Could you check a few things on this model? Use its own coordinates, in mm. Face numbers are marked on the shaded views. A direction names the side the tool comes from. Coordinates: 2 decimals unless noted, no trailing zeros. Loops run counter-clockwise (first coordinate to the right, second up) from the corner with the lowest first, then second, coordinate; pieces in that order, holes last.
1) If I drill on line 1 along X through (y, z) = (8, -12); line 2 along X through (y, z) = (5, -10.5); line 3 along Z through (x, y) = (14, 8.25), over which ranges is the centre line in solid material (lowest first)?
2) Imagine slicing it at C-C on x = -5. Please give me the cut outline in (y, z), plus the area to 3 significant figures.
3) For the marked faces 4 and 5, which set-ups out of +Z, -Z, +X, -X, +Y, -Y let a thin tool reach every point of the face, with its end or its side?
4) Imagine slicing it at B-B on x = -29.8. Please give me the cut outline in (y, z), plus the area to 3 significant figures.
5) Will these pins go through, and if not, where does the flat tip stop? P1, Ø1.4, axis at y = 8, z = -17.5, coming from the -X side; P2, Ø0.9, axis at x = -29.5, y = 1.5, coming from the +Z side; P3, Ø1, axis at x = 2, z = -18, coming from the +Y side.
6) Imagine slicing it at A-A on z = -7.6. Please give me the cut outline in (x, y), plus the area to 3 significant figures.
7) Imagine slicing it at D-D on z = 6.5. Please give me the cut outline in (x, y), plus the area to 3 significant figures.
8) Thinking about a two-plate mould opening in Z: for the marked faces 1, 2 and 3, which applies, released by +Z, released by -Z, zero draft, split by the parting line, or undercut?
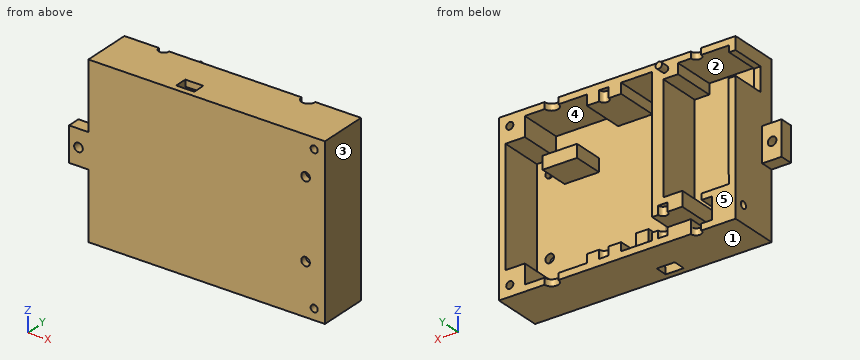
```python
from build123d import *

# Parameters (mm, degrees)
SKETCH_1_W            = 55
SKETCH_1_H            = 39
EXTRUDE_1_DEPTH       = 11.5
SHELL_1_T             = -1.5
SKETCH_2_R            = 1.6
SKETCH_2_R_2          = 1.2
SKETCH_2_W            = 4.2
SKETCH_2_H            = 2.9
CUT_EXTRUDE_1_DEPTH   = 50.086658065
SKETCH_3_W            = 0.1
SKETCH_3_H            = 20.6
SKETCH_3_W_2          = 9
SKETCH_3_H_2          = 1.7
SKETCH_3_W_3          = 8
SKETCH_3_H_3          = 1.95
SKETCH_3_H_4          = 2.4
SKETCH_3_W_4          = 4.5
SKETCH_3_H_5          = 4.5
EXTRUDE_2_DEPTH       = 10
CUT_EXTRUDE_START     = -1.5
SKETCH_4_R            = 1.1
CUT_EXTRUDE_2_DEPTH   = 36
SKETCH_5_R            = 1.1
CUT_EXTRUDE_3_DEPTH   = 7
EXTRUDE_3_DEPTH       = 1.5
EXTRUDE_3_DEPTH_BACK  = 1.5
SKETCH_6_W            = 3
SKETCH_6_H            = 3
SKETCH_6_W_2          = 4.5
SKETCH_6_H_2          = 8
SKETCH_7_R            = 1
SKETCH_7_R_2          = 0.825
CUT_EXTRUDE_4_DEPTH   = 40.198214245
SKETCH_8_R            = 1
CUT_EXTRUDE_5_DEPTH   = 39.784661917
CUT_EXTRUDE_6_REACH   = 61.477
SKETCH_9_R            = 0.825
SKETCH_10_W           = 8
SKETCH_10_H           = 3
F_3MM_4_DEPTH         = 7
CUT_EXTRUDE_4_2_REACH = 61.477
SKETCH_11_W           = 5.5
SKETCH_11_H           = 8
SKETCH_12_R           = 0.75
EXTRUDE_5_DEPTH       = 2


with BuildPart() as part:
    # 草图1 → 凸台-拉伸1 (new body)
    with BuildSketch(Plane(origin=(0, 0, 0), x_dir=(1, 0, 0), z_dir=(0, 1, 0))):
        Rectangle(SKETCH_1_W, SKETCH_1_H)
    extrude(amount=EXTRUDE_1_DEPTH)

    # 抽壳1
    shell_1_openings = [part.faces().sort_by_distance(p)[0] for p in [
        (0, 11.5, 0),
    ]]
    offset(amount=SHELL_1_T, openings=shell_1_openings, kind=Kind.INTERSECTION)

    # 草图2 → 切除-拉伸1 (cut, through all)
    with BuildSketch(Plane(origin=(0, 0, -19.5), x_dir=(-1, 0, 0), z_dir=(0, 0, -1))):
        with Locations((-15.3, 11.5)):
            Circle(SKETCH_2_R)
        with Locations((18.3, 11.5)):
            Circle(SKETCH_2_R_2)
        with Locations((6, 2.85)):
            Rectangle(SKETCH_2_W, SKETCH_2_H)
    extrude(amount=-CUT_EXTRUDE_1_DEPTH, mode=Mode.SUBTRACT)

    # 草图3 → 凸台-拉伸2 (add)
    with BuildSketch(Plane(origin=(0, 1.5, 0), x_dir=(1, 0, 0), z_dir=(0, 1, 0))):
        Polygon((-10.7, 9.6), (-10.7, -15.6), (-14.1, -15.6), (-14.1, -18), (-10.7, -18), (-8.1, -18), (-8.1, 13), (-15.1, 13), (-15.1, 9.6), align=None)
        with Locations((-25.95, -0.7)):
            Rectangle(SKETCH_3_W, SKETCH_3_H)
        with Locations((-12.6, 17.15)):
            Rectangle(SKETCH_3_W_2, SKETCH_3_H_2)
        with Locations((3.1, 17.025)):
            Rectangle(SKETCH_3_W_3, SKETCH_3_H_3)
        with Locations((3.1, -16.8)):
            Rectangle(SKETCH_3_W_3, SKETCH_3_H_4)
        with Locations((23.75, 15.75)):
            Rectangle(SKETCH_3_W_4, SKETCH_3_H_5)
        with Locations((23.75, -15.75)):
            Rectangle(SKETCH_3_W_4, SKETCH_3_H_5)
        Polygon((-26, 18), (-22, 18), (-22, 13), (-19.6, 13), (-19.6, 11.6), (-26, 11.6), (-26, 13), align=None)
    extrude(amount=EXTRUDE_2_DEPTH)

    # 草图4 → 切除-拉伸2 (cut)
    with BuildSketch(Plane.XY.offset(19.5).offset(CUT_EXTRUDE_START)):
        with Locations((3.1, 11.5)):
            Circle(SKETCH_4_R)
    extrude(amount=-CUT_EXTRUDE_2_DEPTH, mode=Mode.SUBTRACT)

    # 草图5 → 切除-拉伸3 (cut)
    with BuildSketch(Plane(origin=(0, 0, -19.5), x_dir=(-1, 0, 0), z_dir=(0, 0, -1)).offset(CUT_EXTRUDE_START)):
        with Locations((10.6, 11.5)):
            Circle(SKETCH_5_R)
    extrude(amount=-CUT_EXTRUDE_3_DEPTH, mode=Mode.SUBTRACT)

    # 草图6 → 变速卡位凸台-拉伸3 (add, two sides: drawn at the far end of the back side and taken through both)
    with BuildSketch(Plane(origin=(0, 1.5, 0), x_dir=(1, 0, 0), z_dir=(0, 1, 0)).offset(-EXTRUDE_3_DEPTH_BACK)):
        with Locations((0.4, 11.1)):
            Rectangle(SKETCH_6_W, SKETCH_6_H)
        with Locations((-29.75, 0)):
            Rectangle(SKETCH_6_W_2, SKETCH_6_H_2)
    extrude(amount=EXTRUDE_3_DEPTH + EXTRUDE_3_DEPTH_BACK)

    # 草图7 → Cut-Extrude 4 (cut, through all)
    with BuildSketch(Plane.XZ):
        with Locations(Location((-29.8, 0, 0), (0, 0, 270))):
            Circle(SKETCH_7_R)
        with Locations(Location((25, 17, 0), (0, 0, 270))):
            Circle(SKETCH_7_R_2)
        with Locations(Location((25, -17, 0), (0, 0, 270))):
            Circle(SKETCH_7_R_2)
    extrude(amount=-CUT_EXTRUDE_4_DEPTH, mode=Mode.SUBTRACT)

    # 草图8 → 底部螺丝孔切除-拉伸5 (cut, through all)
    with BuildSketch(Plane(origin=(0, 1.5, 0), x_dir=(1, 0, 0), z_dir=(0, 1, 0))):
        with Locations(Location((23, 7.6, 0), (0, 0, 270))):
            Circle(SKETCH_8_R)
        with Locations(Location((23, -10.5, 0), (0, 0, 270))):
            Circle(SKETCH_8_R)
    extrude(amount=-CUT_EXTRUDE_5_DEPTH, mode=Mode.SUBTRACT)

    # 草图9 → 前螺丝孔切除-拉伸6 (cut, up to next)
    with BuildSketch(Plane.ZY.offset(27.5), mode=Mode.PRIVATE) as cut_extrude_6_sk1:
        with Locations((-15.501988962, 9)):
            Circle(SKETCH_9_R)
    cut_extrude_6_tool1 = extrude(cut_extrude_6_sk1.sketch, amount=-CUT_EXTRUDE_6_REACH, mode=Mode.PRIVATE) & part.part
    add(cut_extrude_6_tool1.solids().sort_by_distance((-27.5, 9, -15.501989))[0], mode=Mode.SUBTRACT)

    # 草图10 → 3mm轴卡位凸台-拉伸4 (add)
    with BuildSketch(Plane(origin=(0, 1.5, 0), x_dir=(1, 0, 0), z_dir=(0, 1, 0))):
        with Locations((15.55, -8.7)):
            Rectangle(SKETCH_10_W, SKETCH_10_H)
    extrude(amount=F_3MM_4_DEPTH)

    # 草图11 → Cut-Extrude 4 2 (cut, up to next)
    with BuildSketch(Plane.ZY.offset(27.5), mode=Mode.PRIVATE) as cut_extrude_4_2_sk1:
        with Locations((13.75, 7.5)):
            Rectangle(SKETCH_11_W, SKETCH_11_H)
    cut_extrude_4_2_tool1 = extrude(cut_extrude_4_2_sk1.sketch, amount=-CUT_EXTRUDE_4_2_REACH, mode=Mode.PRIVATE) & part.part
    add(cut_extrude_4_2_tool1.solids().sort_by_distance((-27.5, 7.5, 13.75))[0], mode=Mode.SUBTRACT)

    # 草图12 → 凸台-拉伸5 (add)
    with BuildSketch(Plane(origin=(0, 11.5, 0), x_dir=(1, 0, 0), z_dir=(0, 1, 0))):
        with Locations(Location((-11.1, -17.6, 0), (0, 0, 270))):
            Circle(SKETCH_12_R)
    extrude(amount=EXTRUDE_5_DEPTH)


solid = part.part
```
Filled in:
1. line 1: x = -27.5 to -19.6, -15.1 to -8.1, 26 to 27.5
1. line 2: x = -27.5 to -26, -15.1 to -8.1, 26 to 27.5
1. line 3: z = -19.5 to -18, 7.2 to 10.2, 18 to 19.5
2. outline: (0, -19.5) - (1.4, -19.5) - (1.4, 19.5) - (0, 19.5) - close; (4.3, -19.5) - (11.5, -19.5) - (11.5, -18) - (4.3, -18) - close; (4.3, 18) - (11.5, 18) - (11.5, 19.5) - (4.3, 19.5) - close
2. area: 76.2 mm2
3. face 4: +Y
3. face 5: +Z, -Z, +X, -X, +Y
4. outline: (0, -4) - (3, -4) - (3, -1) - (0, -1) - close; (0, 1) - (3, 1) - (3, 4) - (0, 4) - close
4. area: 18.0 mm2
5. P1: stops at x = -27.5
5. P2: stops at z = 4
5. P3: stops at y = 11.5
6. outline: (-27.5, 0) - (22, 0) - (22, 1.5) - (-3.9, 1.5) - (-3.9, 1.4) - (-8.1, 1.4) - (-8.1, 11.5) - (-10.7, 11.5) - (-10.7, 1.5) - (-25.9, 1.5) - (-25.9, 11.5) - (-27.5, 11.5) - close; (24, 0) - (27.5, 0) - (27.5, 11.5) - (26, 11.5) - (26, 1.5) - (24, 1.5) - close
6. area: 136 mm2
7. outline: (-27.5, 0) - (27.5, 0) - (27.5, 11.5) - (26, 11.5) - (26, 1.5) - (-3.9, 1.5) - (-3.9, 1.4) - (-8.1, 1.4) - (-8.1, 11.5) - (-10.7, 11.5) - (-10.7, 1.5) - (-25.9, 1.5) - (-25.9, 11.5) - (-27.5, 11.5) - close
7. area: 139 mm2
8. face 1: released by -Z
8. face 2: undercut
8. face 3: zero draft
